Design review of the part built by this model. Coordinates are the model's own, in mm. Give positions to 0.01 mm unless a question says otherwise; leave off trailing zeros. Order: outer loops, then holes, each group sorted by start corner. A loop starts at its lowest first (then second) coordinate and runs counter-clockwise, first axis right, second up. Notation, with made-up numbers: (37.5, -22) -> (53.5, -22) arc R15 cw to (53.5, -16) -> close; hole circle Ø4 at (30, 31). An arc over 180 degrees is marked (long way). One line per item, written item: value.
from build123d import *

# Parameters (mm, degrees)
SKETCH1_W           = 66.675
SKETCH1_H           = 66.675
SKETCH1_R           = 3.175
SKETCH1_R_2         = 14.3002
SKETCH1_R_3         = 2.1828125
BOSS_EXTRUDE1_DEPTH = 3.175
FILLET1_R           = 3.175


with BuildPart() as part:
    # Sketch1 → Boss-Extrude1 (new body)
    with BuildSketch(Plane(origin=(0, 0, 0), x_dir=(0, 0, -1), z_dir=(1, 0, 0))):
        Rectangle(SKETCH1_W, SKETCH1_H)
        with Locations((-26.870057685, 26.870057685)):
            Circle(SKETCH1_R, mode=Mode.SUBTRACT)
        with Locations((26.870057685, 26.870057685)):
            Circle(SKETCH1_R, mode=Mode.SUBTRACT)
        with Locations((26.870057685, -26.870057685)):
            Circle(SKETCH1_R, mode=Mode.SUBTRACT)
        with Locations((-26.870057685, -26.870057685)):
            Circle(SKETCH1_R, mode=Mode.SUBTRACT)
        Circle(SKETCH1_R_2, mode=Mode.SUBTRACT)
        with Locations((0, 23.8125)):
            Circle(SKETCH1_R_3, mode=Mode.SUBTRACT)
        with Locations((20.622229928, 11.90625)):
            Circle(SKETCH1_R_3, mode=Mode.SUBTRACT)
        with Locations((20.622229928, -11.90625)):
            Circle(SKETCH1_R_3, mode=Mode.SUBTRACT)
        with Locations((0, -23.8125)):
            Circle(SKETCH1_R_3, mode=Mode.SUBTRACT)
        with Locations((-20.622229928, -11.90625)):
            Circle(SKETCH1_R_3, mode=Mode.SUBTRACT)
        with Locations((-20.622229928, 11.90625)):
            Circle(SKETCH1_R_3, mode=Mode.SUBTRACT)
    extrude(amount=BOSS_EXTRUDE1_DEPTH)

    # Fillet1
    fillet1_edges = [part.edges().sort_by_distance(p)[0] for p in [
        (1.5875, -33.3375, -33.3375),
        (1.5875, -33.3375, 33.3375),
        (1.5875, 33.3375, 33.3375),
        (1.5875, 33.3375, -33.3375),
    ]]
    fillet(fillet1_edges, radius=FILLET1_R)


solid = part.part
Item 1: To check wall thickness, follow line 1 along Y through (x, z) = (2.65, 0); line 2 along Z through (x, y) = (2, 27); line 3 along Z through (x, y) = (2.65, 28). State the ranges of each line that lie inside material, in increasing order. Write a range as from..to.
Returned:
line 1: -33.34..-26, -21.63..-14.3, 14.3..21.63, 26..33.34
line 2: -33.34..-30.04, -23.7..23.7, 30.04..33.34
line 3: -33.34..-29.84, -23.9..23.9, 29.84..33.34
Item 2: Draft analysis for pull direction Z (two halves, no side actions). For faces 1 (the flat face through (2, 33.338, 0)), 2 (the cylindrical face through (1.565, -25.749, -1.007)), 3 (the flat face through (2, 0, 33.338)), state which applies: pulls with the +Z half, pulls with the -Z half, needs draft (parallel to the pull), parting line crosses it, or undercut.
Returned:
face 1: needs draft
face 2: undercut
face 3: pulls with the +Z half
Item 3: Add section D-D on z = 26.5. Give the boundary of the cut face in (x, y) (1 decimal).
Returned:
outline: (0, -33.3) -> (3.2, -33.3) -> (3.2, -30) -> (0, -30) -> close; (0, -23.7) -> (3.2, -23.7) -> (3.2, 23.7) -> (0, 23.7) -> close; (0, 30) -> (3.2, 30) -> (3.2, 33.3) -> (0, 33.3) -> close
Item 4: Add section A-A on z = 0. Give the boundary of the cut face in (x, y) (1 decimal), plus the area to 3 significant figures.
Returned:
outline: (0, -33.3) -> (3.2, -33.3) -> (3.2, -26) -> (0, -26) -> close; (0, -21.6) -> (3.2, -21.6) -> (3.2, -14.3) -> (0, -14.3) -> close; (0, 14.3) -> (3.2, 14.3) -> (3.2, 21.6) -> (0, 21.6) -> close; (0, 26) -> (3.2, 26) -> (3.2, 33.3) -> (0, 33.3) -> close
area: 93.2 mm²
Item 5: Add section C-C on z = -11. Give the boundary of the cut face in (x, y) (1 decimal), plus the area to 3 significant figures.
Returned:
outline: (0, -33.3) -> (3.2, -33.3) -> (3.2, -9.1) -> (0, -9.1) -> close; (0, 9.1) -> (3.2, 9.1) -> (3.2, 33.3) -> (0, 33.3) -> close
area: 154 mm²
Item 6: Add section B-B on y = 0. Give the boundary of the cut face in (x, z) (1 decimal), plus the area to 3 significant figures.
Returned:
outline: (0, -33.3) -> (3.2, -33.3) -> (3.2, -14.3) -> (0, -14.3) -> close; (0, 14.3) -> (3.2, 14.3) -> (3.2, 33.3) -> (0, 33.3) -> close
area: 121 mm²
